Check sheet for the modelled part. Datum: model origin and axes. Units: mm. Face numbers are marked on the shaded views. A direction names the side the tool comes from. Round coordinates to 2 decimals unless told otherwise and drop trailing zeros. Write each loop counter-clockwise with the first axis right and the second up, starting at its lowest first coordinate (ties: lowest second). Pieces come first, ordered by that corner, then holes.
Item 1: Depth check by flat-ended pin: pin 1 (6 mm diameter, centred on x = 32.5, y = 19, fed in from +Z); pin 2 (15.5 mm diameter, centred on y = -43, z = -19.5, fed in from +X); pin 3 (24 mm diameter, centred on x = 29.5, z = -15, fed in from -Y); pin 4 (11 mm diameter, centred on x = 74, z = -21.75, fed in from +Y). Enter the tip coordinate at first touch or a pass-through.
Item 2: Set-up check for the marked faces 4, 5, 6 and 7: record each of +Z, -Z, +X, -X, +Y, -Y from which the full face is reachable in a straight line by a thin tool's end or side.
Item 3: Section check D-D, the plane y = 8. Record the cut outline in (x, z).
Item 4: Section check C-C, the plane z = 30. Record the cut outline in (x, y), plus the area to 3 significant figures.
Item 5: Section check A-A, the plane y = 93. Record the cut outline in (x, z).
Item 6: Material ranges on line 1 along X through (y, z) = (-93, -7); line 2 along Y through (x, z) = (0, -23); line 3 along Y through (x, z) = (95.5, -16.5), recorded low to high.
Item 7: Release check for a two-part mould opening along Y. For the marked faces 1, 2 and 3 record: pulls with the +Y half, pulls with the -Y half, needs draft (parallel to the pull), parting line crosses it, or undercut.
Item 8: Section check B-B, the plane x = 59. Record the cut outline in (y, z), plus the area to 3 significant figures.
from build123d import *

# Parameters (mm, degrees)
SKETCH021_R          = 33
PAD012_DEPTH         = 35
PAD012_DEPTH_BACK    = 12.5
PAD013_START         = 12.5
SKETCH022_W          = 44.5
SKETCH022_H          = 210
PAD013_DEPTH         = 25
POCKET005_DEPTH      = 6.5
POCKET005_DEPTH_BACK = 13
SKETCH_2_R           = 6
POCKET006_DEPTH      = 50
POCKET006_DEPTH_BACK = 50
SKETCH028_R          = 6
POCKET011_DEPTH      = 180.001


with BuildPart() as part:
    # Sketch021 → Pad012 (new body, two sides)
    with BuildSketch(Plane.XY) as pad012_sk:
        with BuildLine():
            Line((-110, -105), (110, -105))
            Line((110, -105), (120.90162, -105))
            ThreePointArc((120.90162, -105), (127.335146, -102.335146), (130, -95.90162))
            Line((130, -95.90162), (130, -89.09838))
            ThreePointArc((130, -89.09838), (127.335146, -82.664854), (120.90162, -80))
            Line((120.90162, -80), (119.09838, -80))
            ThreePointArc((110, -70.90162), (112.664854, -77.335146), (119.09838, -80))
            Line((110, -70.90162), (110, 0))
            Line((110, 70.90162), (110, 0))
            ThreePointArc((119.09838, 80), (112.664854, 77.335146), (110, 70.90162))
            Line((120.90162, 80), (119.09838, 80))
            ThreePointArc((120.90162, 80), (127.335146, 82.664854), (130, 89.09838))
            Line((130, 95.90162), (130, 89.09838))
            ThreePointArc((130, 95.90162), (127.335146, 102.335146), (120.90162, 105))
            Line((110, 105), (120.90162, 105))
            Line((110, 105), (-110, 105))
            Line((-110, 105), (-110, 0))
            Line((-110, -105), (-110, 0))
        make_face()
        Circle(SKETCH021_R, mode=Mode.SUBTRACT)
    extrude(amount=-PAD012_DEPTH)
    extrude(pad012_sk.sketch, amount=PAD012_DEPTH_BACK)

    # Sketch022 → Pad013 (join)
    with BuildSketch(Plane.XY.offset(PAD013_START)):
        with Locations((-87.75, 0)):
            Rectangle(SKETCH022_W, SKETCH022_H)
    extrude(amount=PAD013_DEPTH)

    # Sketch_1 → Pocket005 (cut, two sides)
    with BuildSketch(Plane.XY) as pocket005_sk:
        Polygon((145.597992, 65.5), (0, 65.5), (-153.015656, 65.5), (-153.015656, -65.5), (0, -65.5), (145.597992, -65.5), align=None)
    extrude(amount=-POCKET005_DEPTH, mode=Mode.SUBTRACT)
    extrude(pocket005_sk.sketch, amount=POCKET005_DEPTH_BACK, mode=Mode.SUBTRACT)

    # Sketch_2 → Pocket006 (cut, two sides)
    with BuildSketch(Plane.XY) as pocket006_sk:
        with Locations((-118, 93)):
            Circle(SKETCH_2_R)
        with Locations((118, 93)):
            Circle(SKETCH_2_R)
        with Locations((-118, -93)):
            Circle(SKETCH_2_R)
        with Locations((118, -93)):
            Circle(SKETCH_2_R)
        Polygon((-0.25, 33.607407), (-0.25, 47.5), (126.736248, 47.5), (126.736248, 47), (0.25, 47), (0.25, 33.607407), align=None)
        with BuildLine():
            ThreePointArc((86.75, 75), (87.81066, 75.43934), (88.25, 76.5))
            Line((88.25, 105), (88.25, 76.5))
            Line((88.25, 105), (6.75, 105))
            Line((6.75, 105), (6.75, 76.5))
            ThreePointArc((6.75, 76.5), (7.18934, 75.43934), (8.25, 75))
            Line((86.75, 75), (8.25, 75))
        make_face()
        Polygon((-0.067348, -33.607407), (-0.067348, -47.5), (126.736248, -47.5), (126.736248, -47), (0.25, -47), (0.25, -33.607407), align=None)
        with BuildLine():
            ThreePointArc((-88.25, 76.5), (-87.81066, 75.43934), (-86.75, 75))
            Line((-86.75, 75), (-8.25, 75))
            ThreePointArc((-8.25, 75), (-7.18934, 75.43934), (-6.75, 76.5))
            Line((-6.75, 105), (-6.75, 76.5))
            Line((-88.25, 105), (-6.75, 105))
            Line((-88.25, 105), (-88.25, 76.5))
        make_face()
        with BuildLine():
            ThreePointArc((88.25, -76.5), (87.81066, -75.43934), (86.75, -75))
            Line((86.75, -75), (8.25, -75))
            ThreePointArc((8.25, -75), (7.18934, -75.43934), (6.75, -76.5))
            Line((6.75, -105), (6.75, -76.5))
            Line((88.25, -105), (6.75, -105))
            Line((88.25, -105), (88.25, -76.5))
        make_face()
        with BuildLine():
            ThreePointArc((-86.75, -75), (-87.81066, -75.43934), (-88.25, -76.5))
            Line((-88.25, -105), (-88.25, -76.5))
            Line((-88.25, -105), (-6.75, -105))
            Line((-6.75, -105), (-6.75, -76.5))
            ThreePointArc((-6.75, -76.5), (-7.18934, -75.43934), (-8.25, -75))
            Line((-86.75, -75), (-8.25, -75))
        make_face()
    extrude(amount=-POCKET006_DEPTH, mode=Mode.SUBTRACT)
    extrude(pocket006_sk.sketch, amount=POCKET006_DEPTH_BACK, mode=Mode.SUBTRACT)

    # Sketch028 → Pocket011 (cut, through all)
    with BuildSketch(Plane.XZ.offset(75)):
        with Locations((74, -21.75)):
            Circle(SKETCH028_R)
    extrude(amount=-POCKET011_DEPTH, mode=Mode.SUBTRACT)


solid = part.part
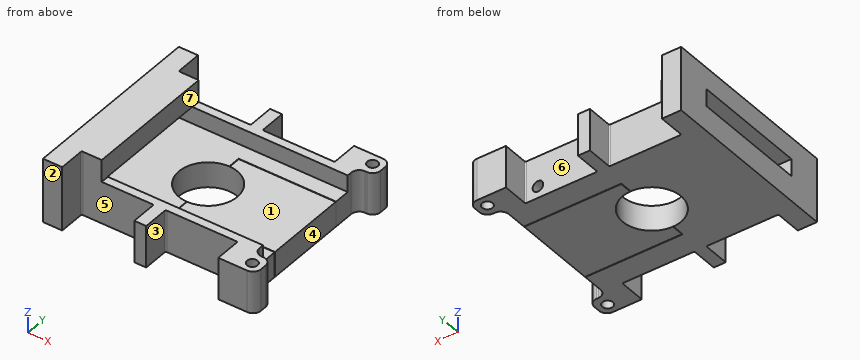
Values found:
1. pin 1: stops at z = -6.5
1. pin 2: stops at x = 110
1. pin 3: stops at y = -75
1. pin 4: passes through
2. face 4: +Z, -Z, +X
2. face 5: +Z, -Z, -Y
2. face 6: +Z, -Z, +Y
2. face 7: +Z, +X, +Y, -Y
3. outline: (-110, -35) - (-32.02, -35) - (-32.02, -6.5) - (-110, -6.5) - close; (-110, 13) - (-65.5, 13) - (-65.5, 37.5) - (-110, 37.5) - close; (32.02, -35) - (110, -35) - (110, -6.5) - (32.02, -6.5) - close; hole circle Ø12 at (74, -21.75)
4. outline: (-110, -105) - (-88.25, -105) - (-88.25, -76.5) arc R1.5 cw to (-86.75, -75) - (-65.5, -75) - (-65.5, 75) - (-86.75, 75) arc R1.5 cw to (-88.25, 76.5) - (-88.25, 105) - (-110, 105) - close
4. area: 7,980 mm2
5. outline: (-110, -35) - (-88.25, -35) - (-88.25, 37.5) - (-110, 37.5) - close; (-6.75, -35) - (6.75, -35) - (6.75, 12.5) - (-6.75, 12.5) - close; (88.25, -35) - (112, -35) - (112, 12.5) - (88.25, 12.5) - close; (124, -35) - (130, -35) - (130, 12.5) - (124, 12.5) - close
6. line 1: x = -110 to -88.25, -6.75 to 6.75, 88.25 to 112, 124 to 130
6. line 2: y = -105 to -47.5, -33.61 to -33, 33 to 33.61, 47.5 to 105
6. line 3: y = -105 to -47.5, -47 to 47, 47.5 to 105
7. face 1: undercut
7. face 2: pulls with the -Y half
7. face 3: needs draft
8. outline: (-75, -35) - (-47.5, -35) - (-47.5, -6.5) - (-65.5, -6.5) - (-65.5, 12.5) - (-75, 12.5) - close; (-47, -35) - (47, -35) - (47, -6.5) - (-47, -6.5) - close; (47.5, -35) - (75, -35) - (75, 12.5) - (65.5, 12.5) - (65.5, -6.5) - (47.5, -6.5) - close
8. area: 4,610 mm2
